Read the model definition and answer for the solid it produces. Units are mm, in the model's axes. A direction names the side the tool comes from. Give positions to 0.01 mm unless a question says otherwise; leave off trailing zeros. Order: outer loops, then holes, each group sorted by start corner. A loop starts at its lowest first (then second) coordinate and runs counter-clockwise, first axis right, second up. Notation, with made-up numbers: (47, 41) - (76, 41) arc R25 ccw to (76, 72) - close; hole circle Ø1 at (-9, 70.25). An arc over 180 degrees is marked (long way). Write each question's results on one line, items separated by ' | '. Start each with the question number.
Q1. A tool of negligible diameter and unlimited length cuts with its end or side. For faces 5 (the face through (-10, -5.08, -2)), 6 (the face through (-17.46, -7.27, 0.14)), from which of +Z, -Z, +X, -X, +Y, -Y can it reach the whole face along a straight path? Write none if from no direction.
Q2. Flat-ended cylindrical pins translate along their axes: P1, Ø2, axis at x = 9.5, z = 3, coming from the +Y side; P2, Ø10, axis at x = 3.5, y = 1, coming from the +Z side; P3, Ø4, axis at x = 11.5, y = 0.5, coming from the -Z side; P4, Ø2, axis at x = -12, y = -4, coming from the -Z side. Find the tip coordinate at first contact, or state that the pin passes through.
Q3. Find the intervals of material crossed by line 1 along Y through (x, z) = (-7, 1) (3 decimals); line 2 along Y through (x, z) = (6.35, 0.05) (3 decimals); line 3 along X through (y, z) = (2, 1), in increasing order. Write a range as from..to.
Q4. Find section A-A on z = 0.5. Give the vertices of the cut face in (x, y) (3 decimals), and give its area (3 significant figures).
Q5. For a pull along Y with two mould halves and no side action, classify faces 1 (the face through (-13.5, 7.3, -0.7)), 2 (the face through (-8, 5.08, 0)), 3 (the face through (-5, -9.525, 0)), 4 (the face through (15.873, 0.209, 0.089)) as +Y half, -Y half, draft (parallel to the pull), parting line (faces both ways), or undercut.
Q6. Find section D-D on z = -1.25. Give the vertices of the cut face in (x, y) (3 decimals).
from build123d import *

# Parameters (mm, degrees)
BOSS_EXTRUDE1_DEPTH         = 9.525
BOSS_EXTRUDE2_DEPTH         = 12.7
CUT_EXTRUDE1_DEPTH          = 5.08
F_10_32_TAPPED_HOLE1_D      = 4.0386
F_10_32_TAPPED_HOLE1_DEPTH  = 4.445
F_10_CLEARANCE_HOLE1_D      = 4.9784
F_10_CLEARANCE_HOLE1_DEPTH  = 14.604
F_1_4_0_25_DIAMETER_HOLE1_D = 6.35
FILLET1_R                   = 6.35


with BuildPart() as part:
    # Sketch1 → Boss-Extrude1 (new, symmetric)
    with BuildSketch(Plane(origin=(0, 0, 0), x_dir=(1, 0, 0), z_dir=(0, 1, 0))):
        with BuildLine():
            Line((0, -6.35), (-11.1125, -6.35))
            ThreePointArc((-11.1125, -6.35), (-17.4625, 0), (-11.1125, 6.35))
            Line((-11.1125, 6.35), (0, 6.35))
            Line((0, 6.35), (0, -6.35))
        make_face()
    extrude(amount=BOSS_EXTRUDE1_DEPTH, both=True)

    # Sketch2 → Boss-Extrude2 (add)
    with BuildSketch(Plane.XY.offset(6.35)):
        with BuildLine():
            Line((0, 9.525), (6.35, 9.525))
            ThreePointArc((6.35, 9.525), (15.875, 0), (6.35, -9.525))
            Line((6.35, -9.525), (0, -9.525))
            ThreePointArc((0, -9.525), (-9.525, 0), (0, 9.525))
        make_face()
    extrude(amount=-BOSS_EXTRUDE2_DEPTH)

    # Sketch3 → Cut-Extrude1 (cut, symmetric)
    with BuildSketch(Plane(origin=(0, 0, 0), x_dir=(1, 0, 0), z_dir=(0, 1, 0))):
        with BuildLine():
            Line((-4.588999966, 6.35), (-11.1125, 6.35))
            ThreePointArc((-11.1125, 6.35), (-17.4625, 0), (-11.1125, -6.35))
            Line((-11.1125, -6.35), (-4.588999966, -6.35))
            Line((-4.588999966, -6.35), (-4.588999966, 6.35))
        make_face()
    extrude(amount=CUT_EXTRUDE1_DEPTH, both=True, mode=Mode.SUBTRACT)

    # #10-32 Tapped Hole1
    with Locations(Plane(origin=(0, -5.08, 0), x_dir=(1, 0, 0), z_dir=(0, 1, 0))):
        with Locations((-11.1125, 0)):
            Hole(F_10_32_TAPPED_HOLE1_D / 2, depth=F_10_32_TAPPED_HOLE1_DEPTH)

    # #10 Clearance Hole1
    with Locations(Plane(origin=(0, 9.525, 0), x_dir=(1, 0, 0), z_dir=(0, 1, 0))):
        with Locations((-11.1125, 0)):
            Hole(F_10_CLEARANCE_HOLE1_D / 2, depth=F_10_CLEARANCE_HOLE1_DEPTH)

    # 1/4 (0.25) Diameter Hole1 (through all)
    with Locations(Plane(origin=(0, 0, -6.35), x_dir=(-1, 0, 0), z_dir=(0, 0, -1))):
        with Locations((-6.35, 0)):
            Hole(F_1_4_0_25_DIAMETER_HOLE1_D / 2)

    # Fillet1
    fillet1_edges = [part.edges().sort_by_distance(p)[0] for p in [
        (3.175, 0, -6.35),
        (3.175, 0, 6.35),
    ]]
    fillet(fillet1_edges, radius=FILLET1_R - 0.0001)  # a hair under: the kernel refuses the full size


solid = part.part
Working result:
1) face 5: +Z, -Z, -X | face 6: -X, +Y, -Y
2) P1: y = 9.28 | P2: z = 6.17 | P3: z = -5.9 | P4: through
3) line 1: -9.525..-5.08, 5.08..9.525 | line 2: -9.525..-3.175, 3.175..9.525 | line 3: -4.59..3.78, 8.92..15.66
4) outline: (-17.443, -9.525) - (-13.069, -9.525) - (-13.069, -5.08) - (-17.443, -5.08) - close; (-17.443, 5.08) - (-13.551, 5.08) - (-13.551, 9.525) - (-17.443, 9.525) - close; (-9.156, -9.525) - (6.35, -9.525) arc R9.525 ccw to (6.35, 9.525) - (-8.674, 9.525) - (-8.674, 5.08) - (-4.589, 5.08) - (-4.589, -5.08) - (-9.156, -5.08) - close; hole circle Ø6.389 at (6.35, 0) | area: 394 mm²
5) face 1: draft | face 2: undercut | face 3: -Y half | face 4: parting line
6) outline: (-17.338, -9.525) - (-12.698, -9.525) - (-12.698, -5.08) - (-17.338, -5.08) - close; (-17.338, 5.08) - (-13.265, 5.08) - (-13.265, 9.525) - (-17.338, 9.525) - close; (-9.527, -9.525) - (6.35, -9.525) arc R9.525 ccw to (6.35, 9.525) - (-8.96, 9.525) - (-8.96, 5.08) - (-4.589, 5.08) - (-4.589, -5.08) - (-9.527, -5.08) - close; hole circle Ø6.598 at (6.35, 0)
